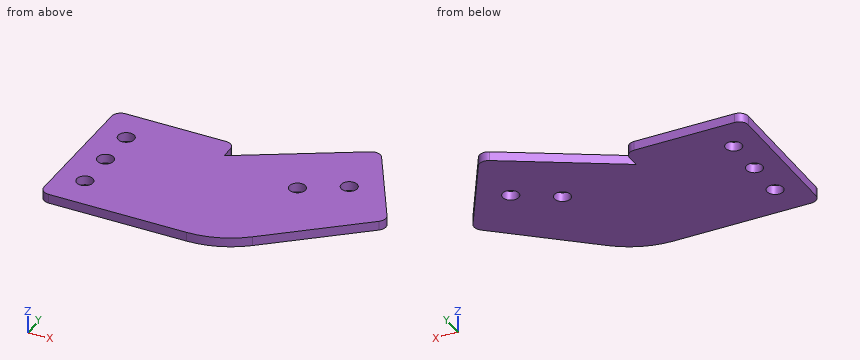
from build123d import *

# Parameters (mm, degrees)
SKETCH1_R           = 1.75
BOSS_EXTRUDE1_DEPTH = 2


with BuildPart() as part:
    # Sketch1 → Boss-Extrude1 (new body)
    with BuildSketch(Plane.XY):
        with BuildLine():
            Line((24.25, 33), (2.5, 33))
            ThreePointArc((2.5, 33), (1.085786438, 32.414213562), (0.5, 31))
            Line((0.5, 31), (0.5, 2.5))
            ThreePointArc((0.5, 2.5), (1.085786438, 1.085786438), (2.5, 0.5))
            Line((2.5, 0.5), (32.377282652, 0.5))
            ThreePointArc((32.377282652, 0.5), (38.790160339, 1.63076336), (44.429550333, 4.886666692))
            Line((44.429550333, 4.886666692), (63.578598927, 20.954626304))
            ThreePointArc((63.578598927, 20.954626304), (64.262639213, 22.139418835), (64.025074515, 23.48671519))
            Line((64.025074515, 23.48671519), (53.513611416, 41.69310334))
            ThreePointArc((53.513611416, 41.69310334), (52.299198698, 42.624954992), (50.781560608, 42.425154147))
            Line((50.781560608, 42.425154147), (26.25, 28.261851027))
            Line((26.25, 28.261851027), (26.25, 31))
            ThreePointArc((26.25, 31), (25.664213562, 32.414213562), (24.25, 33))
        make_face()
        with Locations((52.79293994, 29.441342951)):
            Circle(SKETCH1_R, mode=Mode.SUBTRACT)
        with Locations((44.132685902, 24.441342951)):
            Circle(SKETCH1_R, mode=Mode.SUBTRACT)
        with Locations((6.5, 25.5)):
            Circle(SKETCH1_R, mode=Mode.SUBTRACT)
        with Locations((6.5, 16.75)):
            Circle(SKETCH1_R, mode=Mode.SUBTRACT)
        with Locations((6.5, 8)):
            Circle(SKETCH1_R, mode=Mode.SUBTRACT)
    extrude(amount=BOSS_EXTRUDE1_DEPTH)


solid = part.part
Part model, mm, in its own coordinate system. Give positions to 0.01 mm unless a question says otherwise; leave off trailing zeros. Write each loop counter-clockwise with the first axis right and the second up, starting at its lowest first coordinate (ties: lowest second). Pieces come first, ordered by that corner, then holes.
1) Pin check, flat tips, straight feed: pin 1 (2 mm diameter, centred on x = 52.79, y = 29.44, fed in from -Z); pin 2 (1 mm diameter, centred on x = 40, z = 1, fed in from -Y); pin 3 (0.6 mm diameter, centred on y = 29.5, z = 1, fed in from +X). Stop position of each tip, or through.
Resolved:
pin 1: passes through
pin 2: stops at y = 1.91
pin 3: stops at x = 60.73
2) Cut at A-A on x = 6.5. Write the cut outline in (y, z), then the cut area to 3 significant figures.
Resolved:
outline: (0.5, 0) - (6.25, 0) - (6.25, 2) - (0.5, 2) - close; (9.75, 0) - (15, 0) - (15, 2) - (9.75, 2) - close; (18.5, 0) - (23.75, 0) - (23.75, 2) - (18.5, 2) - close; (27.25, 0) - (33, 0) - (33, 2) - (27.25, 2) - close
area: 44.0 mm2
3) Cut at C-C on z = 1.45. Write the cut outline in (x, y).
Resolved:
outline: (0.5, 2.5) arc R2 ccw to (2.5, 0.5) - (32.38, 0.5) arc R18.75 ccw to (44.43, 4.89) - (63.58, 20.95) arc R2 ccw to (64.03, 23.49) - (53.51, 41.69) arc R2 ccw to (50.78, 42.43) - (26.25, 28.26) - (26.25, 31) arc R2 ccw to (24.25, 33) - (2.5, 33) arc R2 ccw to (0.5, 31) - close; hole circle Ø3.5 at (6.5, 8); hole circle Ø3.5 at (6.5, 16.75); hole circle Ø3.5 at (6.5, 25.5); hole circle Ø3.5 at (44.13, 24.44); hole circle Ø3.5 at (52.79, 29.44)
4) Cut at B-B on y = 16.75. Write the cut outline in (x, z).
Resolved:
outline: (0.5, 0) - (4.75, 0) - (4.75, 2) - (0.5, 2) - close; (8.25, 0) - (58.57, 0) - (58.57, 2) - (8.25, 2) - close
5) Cut at D-D on y = 25.5. Write the cut outline in (x, z).
Resolved:
outline: (0.5, 0) - (4.75, 0) - (4.75, 2) - (0.5, 2) - close; (8.25, 0) - (42.74, 0) - (42.74, 2) - (8.25, 2) - close; (45.53, 0) - (62.86, 0) - (62.86, 2) - (45.53, 2) - close
6) Probe L1, parallel to Y at x = 6.5, z = 0.55; L2, parallel to Y at x = 17.5, z = 0.9; L3, parallel to X at y = 24, z = 0.65. List the from-to ranges inside material, lowest first.
Resolved:
L1: y = 0.5 to 6.25, 9.75 to 15, 18.5 to 23.75, 27.25 to 33
L2: y = 0.5 to 33
L3: x = 0.5 to 5.6, 7.4 to 42.44, 45.83 to 63.73
